Autodesk Inventor part; units mm, degrees
ref_plane "YZ Plane" through (0, 0, 0) normal (1, 0, 0) x (0, 1, 0)
ref_plane "XZ Plane" through (0, 0, 0) normal (0, 1, 0) x (-1, 0, 0)
ref_plane "XY Plane" through (0, 0, 0) normal (0, 0, 1) x (1, 0, 0)
sketch "Sketch2" plane through (0, 0, 0) normal (0, 0, 1) x (1, 0, 0)
  line L0 (-46, 11.5) -> (46, 11.5)
  line L1 (47, 10.5) -> (47, -10.5)
  line L2 (46, -11.5) -> (-46, -11.5)
  line L3 (-47, -10.5) -> (-47, 10.5)
  line L4 (-47, 11.5) -> (47, -11.5) construction
  line L5 (47, 11.5) -> (-47, -11.5) construction
  line L6 (48, 12.5) -> (-48, 12.5)
  line L7 (-48, 12.5) -> (-48, -12.5)
  line L8 (-48, -12.5) -> (48, -12.5)
  line L9 (48, -12.5) -> (48, 12.5)
  arc A0 (47, 10.5) -> (46, 11.5) centre (46, 10.5) ccw
  arc A1 (46, -11.5) -> (47, -10.5) centre (46, -10.5) ccw
  arc A2 (-47, -10.5) -> (-46, -11.5) centre (-46, -10.5) ccw
  arc A3 (-46, 11.5) -> (-47, 10.5) centre (-46, 10.5) ccw
  line L10 (-45, -6.5) -> (45, -6.5)
  line L11 (45, -6.5) -> (45, 9.5)
  line L12 (45, 9.5) -> (-45, 9.5)
  line L13 (-45, 9.5) -> (-45, -6.5)
  point P0 (0, 0)
  point P1 (0, 1.6851)
  dimension "d0" = 94
  dimension "d1" = 23
  dimension "d3" = 1
  dimension "d10" = 1
  dimension "d84" = 90
  dimension "d85" = 16
  dimension "d86" = 2
  dimension "d87" = 2
  dimension "d95" = 2
extrude "Extrusion1" add sketch "Sketch2" along normal blind 1 contours L0 A0 L1 A1 L2 A2 L3 A3 | L9 L8 L7 L6 | L13 L12 L11 L10
extrude "Extrusion2" add sketch "Sketch2" along normal blind 7 contours L9 L8 L7 L6
extrude "Extrusion3" add sketch "Sketch2" along normal blind 4 contours L13 L12 L11 L10
sketch "Sketch4" plane through (-48, -12.5, 0) normal (0, -1, 0) x (1, 0, 0)
  circle A0 centre (22.1132, 5) radius 0.5
  circle A1 centre (29.8868, 5) radius 0.5
  circle A2 centre (44.1132, 5) radius 0.5
  circle A3 centre (51.8842, 5) radius 0.5
  circle A4 centre (66.1132, 5) radius 0.5
  circle A5 centre (73.8868, 5) radius 0.5
  line L0 (0, 6) -> (96, 6)
  line L1 (96, 7) -> (0, 7)
  line L2 (22.1132, 2) -> (22.1132, 2)
  line L3 (22.6132, 2.5) -> (22.6132, 8)
  line L4 (22.6132, 8) -> (21.6132, 8)
  line L5 (21.6132, 8) -> (21.6132, 2.5)
  line L6 (21.6132, 2) -> (22.6132, 8) construction
  line L7 (22.6132, 2) -> (21.6132, 8) construction
  line L8 (29.8868, 2) -> (29.8868, 2)
  line L9 (30.3868, 2.5) -> (30.3868, 8)
  line L10 (30.3868, 8) -> (29.3868, 8)
  line L11 (29.3868, 8) -> (29.3868, 2.5)
  line L12 (29.3868, 2) -> (30.3868, 8) construction
  line L13 (30.3868, 2) -> (29.3868, 8) construction
  line L14 (44.1132, 2) -> (44.1132, 2)
  line L15 (44.6132, 2.5) -> (44.6132, 8)
  line L16 (44.6132, 8) -> (43.6132, 8)
  line L17 (43.6132, 8) -> (43.6132, 2.5)
  line L18 (43.6132, 2) -> (44.6132, 8) construction
  line L19 (44.6132, 2) -> (43.6132, 8) construction
  line L20 (51.8842, 2) -> (51.8842, 2)
  line L21 (52.3842, 2.5) -> (52.3842, 8)
  line L22 (52.3842, 8) -> (51.3842, 8)
  line L23 (51.3842, 8) -> (51.3842, 2.5)
  line L24 (51.3842, 2) -> (52.3842, 8) construction
  line L25 (52.3842, 2) -> (51.3842, 8) construction
  line L26 (66.1132, 2) -> (66.1132, 2)
  line L27 (65.6132, 2.5) -> (65.6132, 8)
  line L28 (65.6132, 8) -> (66.6132, 8)
  line L29 (66.6132, 8) -> (66.6132, 2.5)
  line L30 (66.6132, 2) -> (65.6132, 8) construction
  line L31 (65.6132, 2) -> (66.6132, 8) construction
  line L32 (73.8868, 2) -> (73.8868, 2)
  line L33 (73.3868, 2.5) -> (73.3868, 8)
  line L34 (73.3868, 8) -> (74.3868, 8)
  line L35 (74.3868, 8) -> (74.3868, 2.5)
  line L36 (74.3868, 2) -> (73.3868, 8) construction
  line L37 (73.3868, 2) -> (74.3868, 8) construction
  arc A6 (21.6132, 2.5) -> (22.1132, 2) centre (22.1132, 2.5) ccw
  arc A7 (22.1132, 2) -> (22.6132, 2.5) centre (22.1132, 2.5) ccw
  arc A8 (29.3868, 2.5) -> (29.8868, 2) centre (29.8868, 2.5) ccw
  arc A9 (29.8868, 2) -> (30.3868, 2.5) centre (29.8868, 2.5) ccw
  arc A10 (43.6132, 2.5) -> (44.1132, 2) centre (44.1132, 2.5) ccw
  arc A11 (44.1132, 2) -> (44.6132, 2.5) centre (44.1132, 2.5) ccw
  arc A12 (51.3842, 2.5) -> (51.8842, 2) centre (51.8842, 2.5) ccw
  arc A13 (51.8842, 2) -> (52.3842, 2.5) centre (51.8842, 2.5) ccw
  arc A14 (65.6132, 2.5) -> (66.1132, 2) centre (66.1132, 2.5) ccw
  arc A15 (66.1132, 2) -> (66.6132, 2.5) centre (66.1132, 2.5) ccw
  arc A16 (73.3868, 2.5) -> (73.8868, 2) centre (73.8868, 2.5) ccw
  arc A17 (73.8868, 2) -> (74.3868, 2.5) centre (73.8868, 2.5) ccw
  point P0 (96, 0)
  point P1 (69, 6)
  point P2 (71, 6)
  point P3 (49, 6)
  point P4 (47, 6)
  point P5 (27, 6)
  point P6 (25, 6)
  point P7 (73.8868, 2)
  point P8 (66.1132, 2)
  point P9 (51.8842, 2)
  point P10 (44.1132, 2)
  point P11 (29.8868, 2)
  point P12 (22.1132, 2)
  dimension "d59" = 1
  dimension "d60" = 1
  dimension "d61" = 1
  dimension "d62" = 1
  dimension "d63" = 1
  dimension "d64" = 1
  dimension "d65" = 1
  dimension "d66" = 6
  dimension "d67" = 1
  dimension "d68" = 6
  dimension "d69" = 1
  dimension "d70" = 6
  dimension "d71" = 1
  dimension "d72" = 6
  dimension "d73" = 1
  dimension "d74" = 6
  dimension "d75" = 1
  dimension "d76" = 6
  dimension "d81" = 0.5
sketch "Sketch3" plane through (0, -12.5, 4) normal (0, -1, 0) x (1, 0, 0)
  line L0 (-53.1158, -2.5) -> (46.8842, -2.5) construction
  line L1 (43, -1.5) -> (23, -1.5) construction
  line L2 (23, -1.5) -> (23, 3.5) construction
  line L3 (23, 3.5) -> (43, 3.5) construction
  line L4 (43, 3.5) -> (43, -1.5) construction
  line L5 (23, -1.5) -> (23, 3.7137) construction
  line L6 (43, -1.5) -> (40.1132, 3.5) construction
  line L7 (46.8842, -2.5) -> (46.8842, 3.2735) construction
  line L8 (23, -1.5) -> (25.8868, 3.5) construction
  line L9 (23, -1.5) -> (23, 3.1279) construction
  line L10 (21, -1.5) -> (18.1132, 3.5) construction
  line L11 (1, 3.5) -> (21, 3.5) construction
  line L12 (1, -1.5) -> (3.8868, 3.5) construction
  line L13 (-1, -1.5) -> (-3.8868, 3.5) construction
  line L14 (-21, 3.5) -> (-1, 3.5) construction
  line L15 (-21, -1.5) -> (-18.1132, 3.5) construction
  line L16 (-23, -1.5) -> (-25.8868, 3.5) construction
  line L17 (-43, 3.5) -> (-23, 3.5) construction
  line L18 (-43, -1.5) -> (-40.1132, 3.5) construction
  line L19 (43, 3.5) -> (-43, 3.5) construction
  line L20 (0, 3.5) -> (0, 3.5) construction
  circle A0 centre (-25.8868, -1.5) radius 0.3
  circle A1 centre (-18.1132, -1.5) radius 0.3
  circle A2 centre (-3.8868, -1.5) radius 0.3
  circle A3 centre (3.8842, -1.5) radius 0.3
  circle A4 centre (18.1132, -1.5) radius 0.3
  circle A5 centre (25.8868, -1.5) radius 0.3
  line L21 (-45, 0) -> (-45, 0)
  line L22 (45, 0) -> (45, 0)
  line L23 (-48, -4) -> (-48, -4)
  line L24 (-48, -1.5) -> (48, -1.5)
  line L25 (48, -4) -> (48, -4)
  line L26 (48, -4) -> (48, 3)
  point P0 (3.8842, 2.5)
  point P1 (25.8868, -1.5)
  point P2 (48, -0.5)
  dimension "d45" = 20
  dimension "d46" = 5
  dimension "d47" = 30
  dimension "d48" = 30
  dimension "d49" = 22
  dimension "d52" = 0
  dimension "d53" = 0.6
  dimension "d54" = 0.6
  dimension "d55" = 0.6
  dimension "d56" = 0.6
  dimension "d57" = 0.6
  dimension "d58" = 0.6
  dimension "d82" = 1
extrude "Extrusion4" [suppressed]
extrude "Extrusion5" cut sketch "Sketch3" against normal blind 15
sketch "Sketch5" plane through (-48, -12.5, 0) normal (-1, 0, 0) x (0, 0, 1)
  line L0 (7, 1) -> (1, 1)
  line L1 (1, 1) -> (1, 6)
  line L2 (1, 6) -> (7, 6)
  line L3 (7, 6) -> (7, 1)
  circle A0 centre (2.5, 3.5) radius 0.75
  point P0 (0, 12.5)
  dimension "d88" = 1.5
  dimension "d89" = 1.5
  dimension "d90" = 2.5
extrude "Extrusion6" cut sketch "Sketch5" against normal blind 2 contours A0
extrude "Extrusion7" add sketch "Sketch3" against normal blind 1
properties part number "sdm_finger_eit_chamber_mould_horizontal_e_holes_v2"
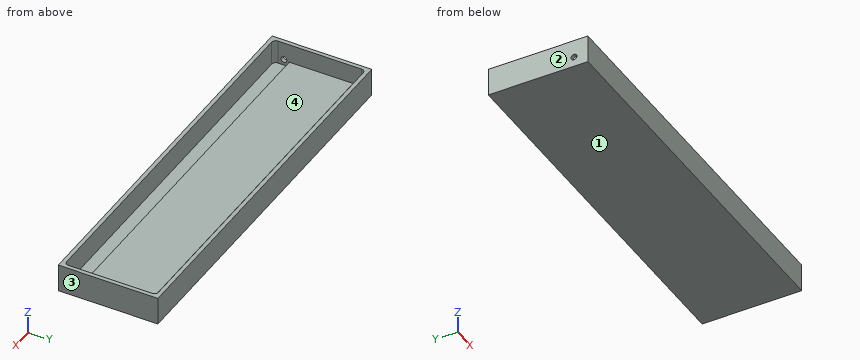
Work out the finished part from the listing and answer in its coordinate system (mm). Face numbers are marked on the shaded views. Coordinates: 2 decimals unless noted, no trailing zeros. Write each loop counter-clockwise with the first axis right and the second up, starting at its lowest first coordinate (ties: lowest second). Pieces come first, ordered by that corner, then holes.
1. The part is cut by section B-B, the plane x = -39.5. Write down the section's boundary in (y, z), and give its area (3 significant figures).
Results list:
outline: (-12.5, 0) - (12.5, 0) - (12.5, 7) - (11.5, 7) - (11.5, 1) - (9.5, 1) - (9.5, 4) - (-6.5, 4) - (-6.5, 1) - (-11.5, 1) - (-11.5, 7) - (-12.5, 7) - close
area: 85.0 mm2
2. For a pull along X with two mould halves and no side action, classify the marked faces 1, 2, 3 and 4 as +X half, -X half, draft (parallel to the pull), parting line (faces both ways), or undercut.
Results list:
face 1: draft
face 2: -X half
face 3: +X half
face 4: undercut
3. The part is cut by section A-A, the plane y = 4.5. Write down the section's boundary in (x, z).
Results list:
outline: (-48, 0) - (48, 0) - (48, 7) - (47, 7) - (47, 1) - (45, 1) - (45, 4) - (-45, 4) - (-45, 1) - (-47, 1) - (-47, 7) - (-48, 7) - close
4. Consider line 1 along Y through (x, z) = (9, 3.25); line 2 along X through (y, z) = (0.75, 1.5); line 3 along X through (y, z) = (-1.75, 6.75). Determine where each line is inside the solid, lowest interval first.
Results list:
line 1: y = -12.5 to -11.5, -6.5 to 9.5, 11.5 to 12.5
line 2: x = -48 to -47, -45 to 45, 47 to 48
line 3: x = -48 to -47, 47 to 48
5. A flat-ended cylindrical pin translates along its axis: pin 1 (13 mm diameter, centred on x = -17, y = -0.5, fed in from +Z). Find the tip coordinate at first contact, or state that the pin passes through.
Results list:
pin 1: stops at z = 4
